Answer from the drawing. Dimensions are ordinates in mm from the lowest x, y and z of the part. A direction names the side the tool comes from. Round coordinates to 2 decimals unless told otherwise and drop trailing zeros. Order: outer loops, then holes, each group sorted by start corner. A loop starts at its lowest first (then second) coordinate and runs counter-clockwise, first axis right, second up. Notation, with made-up numbers: M 68,-16.5 L 79,-16.5 A27 ccw 79,6.5 Z; hole C -24,28.5 d4. An arc over 180 degrees is marked long. Answer as a JSON object with one key per item and string values. Group by question number.
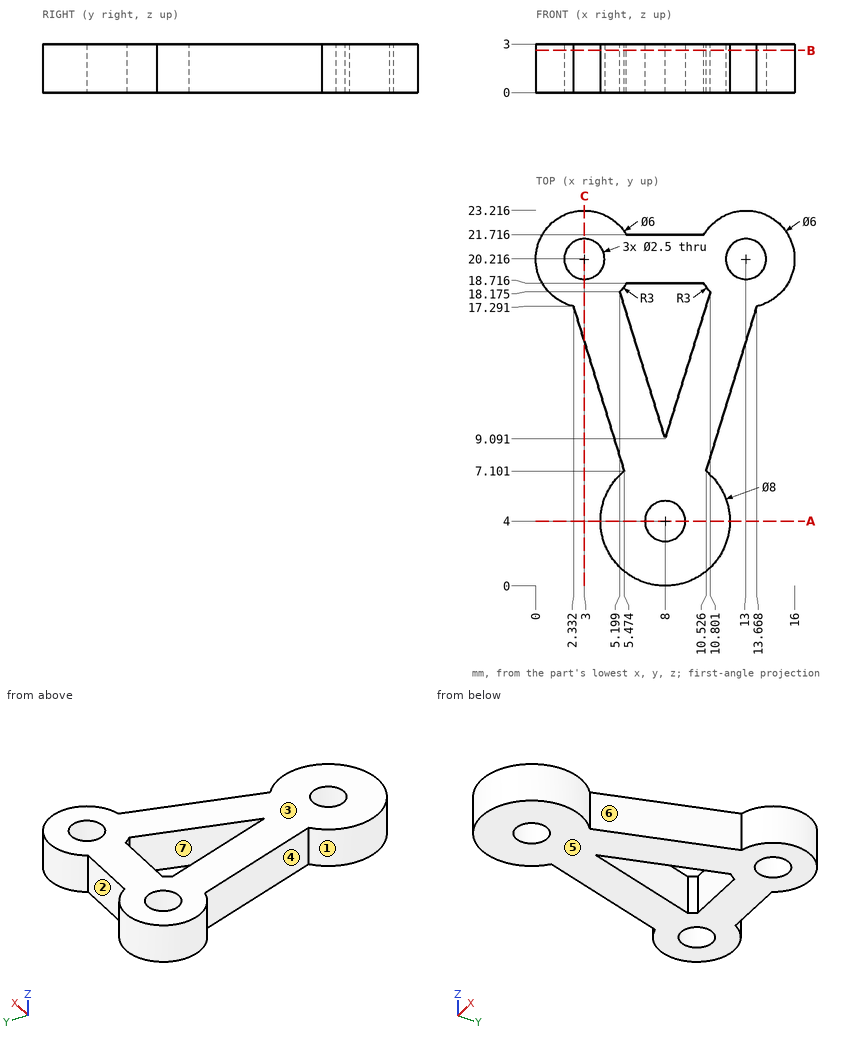
Item 1: The mould has two halves that part along X. Classify the marked faces 1, 2 and 3: +X half, -X half, draft (parallel to the pull), parting line (faces both ways), or undercut.
Item 2: Each of these flat-tipped pins is pushed along its axis until it touches: pin 1 (1 mm diameter, centred on y = 13, z = 2, fed in from +X); pin 2 (2 mm diameter, centred on x = 13, y = 20.22, fed in from +Z); pin 3 (1 mm diameter, centred on x = 11.5, z = 1, fed in from +Y); pin 4 (1.5 mm diameter, centred on x = 8, z = 1, fed in from +Y) (1 decimal). Where does it stop, or does it pass through?
Item 3: Find section A-A (y = 4). Give the vertices of the cut face in (x, z), and give its area (3 significant figures).
Item 4: Consider L1, parallel to X at y = 20.25, z = 0.9; L2, parallel to X at y = 21, z = 1.7 (1 decimal); L3, parallel to X at y = 13.5, z = 2.65. Determine where each line is inside the solid, lowest interval first.
Item 5: A tool of negligible diameter and unlimited length cuts with its end or side. For the marked faces 4, 5, 6 and 7, from which of +Z, -Z, +X, -X, +Y, -Y can it reach the whole face along a straight path? Write none if from no direction.
Item 6: Find section C-C (x = 3). Give the vertices of the cut face in (y, z) (1 decimal).
Item 7: Find section B-B (z = 2.6). Give the number of separate pieces and of enclosed holes in the cut face, and give its area (3 significant figures).
Responses:
{
 "1": {"face 1": "parting line", "face 2": "undercut", "face 3": "draft"},
 "2": {"pin 1": "stops at x = 12.5", "pin 2": "passes through", "pin 3": "stops at y = 23.04", "pin 4": "stops at y = 21.7"},
 "3": {"outline": "M 4,0 L 6.75,0 L 6.75,3 L 4,3 Z; M 9.25,0 L 12,0 L 12,3 L 9.25,3 Z", "area": "16.5 mm^2"},
 "4": {"L1": "x = 0 to 1.75, 4.25 to 11.75, 14.25 to 16", "L2": "x = 0.1 to 2, 4 to 12, 14 to 15.9", "L3": "x = 3.5 to 6.64, 9.36 to 12.5"},
 "5": {"face 4": "+Z, -Z, -X", "face 5": "-Z, +X, -X, +Y, -Y", "face 6": "+Z, -Z, +X", "face 7": "+Z, -Z"},
 "6": {"outline": "M 15.1,0 L 19,0 L 19,3 L 15.1,3 Z; M 21.5,0 L 23.2,0 L 23.2,3 L 21.5,3 Z"},
 "7": {"separate pieces": "1", "enclosed holes": "4", "area": "166 mm^2"}
}
